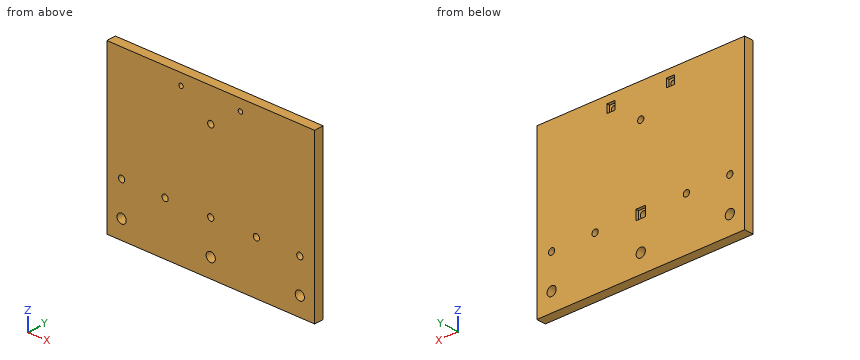
from build123d import *

# Parameters (mm, degrees)
SKETCH2_W           = 140
SKETCH2_H           = 110
SKETCH2_R           = 2.1
SKETCH2_R_2         = 3.1
SKETCH2_R_3         = 1.5
BOSS_EXTRUDE2_DEPTH = 6.35
SKETCH3_W           = 6.5
SKETCH3_H           = 6.5
SKETCH3_W_2         = 5.5
SKETCH3_H_2         = 5.5
CUT_EXTRUDE1_DEPTH  = 2


with BuildPart() as part:
    # Sketch2 → Boss-Extrude2 (new body)
    with BuildSketch(Plane(origin=(0, 0, 0), x_dir=(1, 0, 0), z_dir=(0, 1, 0))):
        with Locations((70, 55)):
            Rectangle(SKETCH2_W, SKETCH2_H)
        with Locations(Location((39.25, 75, 0), (0, 0, 270))):
            Circle(SKETCH2_R, mode=Mode.SUBTRACT)
        with Locations(Location((100.75, 75, 0), (0, 0, 270))):
            Circle(SKETCH2_R, mode=Mode.SUBTRACT)
        with Locations(Location((70, 22, 0), (0, 0, 270))):
            Circle(SKETCH2_R, mode=Mode.SUBTRACT)
        with Locations(Location((10, 97.5, 0), (0, 0, 270))):
            Circle(SKETCH2_R_2, mode=Mode.SUBTRACT)
        with Locations(Location((70, 97.5, 0), (0, 0, 270))):
            Circle(SKETCH2_R_2, mode=Mode.SUBTRACT)
        with Locations(Location((130, 97.5, 0), (0, 0, 270))):
            Circle(SKETCH2_R_2, mode=Mode.SUBTRACT)
        with Locations(Location((10, 75, 0), (0, 0, 270))):
            Circle(SKETCH2_R, mode=Mode.SUBTRACT)
        with Locations(Location((70, 75, 0), (0, 0, 270))):
            Circle(SKETCH2_R, mode=Mode.SUBTRACT)
        with Locations(Location((130, 75, 0), (0, 0, 270))):
            Circle(SKETCH2_R, mode=Mode.SUBTRACT)
        with Locations(Location((50, 7.5, 0), (0, 0, 270))):
            Circle(SKETCH2_R_3, mode=Mode.SUBTRACT)
        with Locations(Location((90, 7.5, 0), (0, 0, 270))):
            Circle(SKETCH2_R_3, mode=Mode.SUBTRACT)
    extrude(amount=BOSS_EXTRUDE2_DEPTH)

    # Sketch3 → Cut-Extrude1 (cut)
    with BuildSketch(Plane(origin=(0, 6.35, 0), x_dir=(1, 0, 0), z_dir=(0, 1, 0))):
        with Locations((70, 75)):
            Rectangle(SKETCH3_W, SKETCH3_H)
        with Locations((50, 7.5)):
            Rectangle(SKETCH3_W_2, SKETCH3_H_2)
        with Locations((90, 7.5)):
            Rectangle(SKETCH3_W_2, SKETCH3_H_2)
    extrude(amount=-CUT_EXTRUDE1_DEPTH, mode=Mode.SUBTRACT)


solid = part.part
Source: CAD feature listing. Evaluate the final solid. Frame: model axes, mm. Give positions to 0.01 mm unless a question says otherwise; leave off trailing zeros. Write each loop counter-clockwise with the first axis right and the second up, starting at its lowest first coordinate (ties: lowest second). Pieces come first, ordered by that corner, then holes. Notation, with made-up numbers: M 82.25,69.5 L 122.25,69.5 A32 ccw 122.25,99.5 Z; hole C 39.5,37.25 d7. An arc over 180 degrees is marked long. Return JSON: item names as keys, results as strings. Group by question number.
1) First-contact query: pin 1 Ø4 at (x, z) = (130, -75) entering from +Y; pin 2 Ø5 at (x, z) = (90, -7.5) entering from +Y. Flat tips, straight axial feed; report the tip coordinate or a pass-through.
2) Cut plane B-B, the plane x = 50. Output: boundary loops of the cut face in (y, z).
3) Cut plane A-A, the plane z = -7.5. Output: boundary loops of the cut face in (x, y).
4) Cut plane D-D, the plane x = 130. Output: boundary loops of the cut face in (y, z), then the cut area to 3 significant figures.
5) Ray query, L1, parallel to X at y = 3.5, z = -75; L2, parallel to X at y = 4.5, z = -6.5; L3, parallel to Z at x = 90, y = 1.1. Return the intervals inside material, ascending.
6) Cut plane C-C, the plane z = -22. Output: boundary loops of the cut face in (x, y).
Data:
{
 "1": {"pin 1": "passes through", "pin 2": "stops at y = 4.35"},
 "2": {"outline": "M 0,-110 L 6.35,-110 L 6.35,-10.25 L 4.35,-10.25 L 4.35,-9 L 0,-9 Z; M 0,-6 L 4.35,-6 L 4.35,-4.75 L 6.35,-4.75 L 6.35,0 L 0,0 Z"},
 "3": {"outline": "M 0,0 L 48.5,0 L 48.5,4.35 L 47.25,4.35 L 47.25,6.35 L 0,6.35 Z; M 51.5,0 L 88.5,0 L 88.5,4.35 L 87.25,4.35 L 87.25,6.35 L 52.75,6.35 L 52.75,4.35 L 51.5,4.35 Z; M 91.5,0 L 140,0 L 140,6.35 L 92.75,6.35 L 92.75,4.35 L 91.5,4.35 Z"},
 "4": {"outline": "M 0,-110 L 6.35,-110 L 6.35,-100.6 L 0,-100.6 Z; M 0,-94.4 L 6.35,-94.4 L 6.35,-77.1 L 0,-77.1 Z; M 0,-72.9 L 6.35,-72.9 L 6.35,0 L 0,0 Z", "area": "632 mm²"},
 "5": {"L1": "x = 0 to 7.9, 12.1 to 37.15, 41.35 to 67.9, 72.1 to 98.65, 102.85 to 127.9, 132.1 to 140", "L2": "x = 0 to 47.25, 52.75 to 87.25, 92.75 to 140", "L3": "z = -110 to -9, -6 to 0"},
 "6": {"outline": "M 0,0 L 67.9,0 L 67.9,6.35 L 0,6.35 Z; M 72.1,0 L 140,0 L 140,6.35 L 72.1,6.35 Z"}
}
